```python
from build123d import *

# Parameters (mm, degrees)
F0_W      = 200
F0_H      = 100
F1_DEPTH  = 20
F3_DEPTH  = 10
F5_DEPTH  = 10
F6_R      = 45
F6_R_2    = 30
F7_DEPTH  = 10
F8_R      = 5
F9_DEPTH  = 25
F10_R     = 30
F11_DEPTH = 22


with BuildPart() as f1:
    # F0 (on Front) → F1 (new body)
    with BuildSketch(Plane.XZ):
        Rectangle(F0_W, F0_H)
    extrude(amount=F1_DEPTH)

    # F2 (on face) → F3 (cut)
    with BuildSketch(Plane.XZ.offset(20)):
        with BuildLine():
            Line((-72, 40), (-78, 40))
            ThreePointArc((-78, 40), (-86.485281, 36.485281), (-90, 28))
            Line((-90, 28), (-90, -28))
            ThreePointArc((-90, -28), (-86.485281, -36.485281), (-78, -40))
            Line((-78, -40), (-72, -40))
            ThreePointArc((-72, -40), (-63.514719, -36.485281), (-60, -28))
            Line((-60, -28), (-60, 28))
            ThreePointArc((-60, 28), (-63.514719, 36.485281), (-72, 40))
        make_face()
    extrude(amount=-F3_DEPTH, mode=Mode.SUBTRACT)

    # F4 (on face) → F5 (join)
    with BuildSketch(Plane.XZ.offset(20)):
        with BuildLine():
            Line((-38, -48), (43.029173, -48))
            ThreePointArc((43.029173, -48), (47.621583, -47.086468), (51.514773, -44.484963))
            Line((51.514773, -44.484963), (85.390988, -10.606203))
            ThreePointArc((85.390988, -10.606203), (89.783988, 0), (85.390988, 10.606203))
            Line((85.390988, 10.606203), (51.514773, 44.484963))
            ThreePointArc((51.514773, 44.484963), (47.621583, 47.086468), (43.029173, 48))
            Line((43.029173, 48), (-38, 48))
            ThreePointArc((-38, 48), (-45.071068, 45.071068), (-48, 38))
            Line((-48, 38), (-48, -38))
            ThreePointArc((-48, -38), (-45.071068, -45.071068), (-38, -48))
        make_face()
    extrude(amount=F5_DEPTH)

    # F6 (on face) → F7 (join)
    with BuildSketch(Plane.XZ.offset(30)):
        Circle(F6_R)
        Circle(F6_R_2, mode=Mode.SUBTRACT)
    extrude(amount=F7_DEPTH)

    # F8 (on face) → F9 (cut)
    with BuildSketch(Plane.XZ.offset(40)):
        with Locations((-37.533723, 0.141637)):
            Circle(F8_R)
        with Locations((36.967181, 0.42491)):
            Circle(F8_R)
        with Locations((0, 37.5)):
            Circle(F8_R)
        with Locations((0.424909, -37.250452)):
            Circle(F8_R)
    extrude(amount=-F9_DEPTH, mode=Mode.SUBTRACT)

    # F10 (on face) → F11 (cut)
    with BuildSketch(Plane.XZ.offset(30)):
        Circle(F10_R)
    extrude(amount=-F11_DEPTH, mode=Mode.SUBTRACT)


solid = f1.part
```
Geometry: final body of the model. Coordinates: model frame, mm. A direction names the side the tool comes from. Give positions to 0.01 mm unless a question says otherwise; leave off trailing zeros. Loops run counter-clockwise (first coordinate to the right, second up) from the corner with the lowest first, then second, coordinate; pieces in that order, holes last. Notation, with made-up numbers: (72.5, -27) - (111.5, -27) arc R33 cw to (111.5, 11) - close; hole circle Ø1 at (-10, -15.75). An arc over 180 degrees is marked (long way). Answer as CSV lines item,"result". Start each with the question number.
(1) Mould query, pull axis X, two halves, no side actions, for faces 4 (the face through (0, -8, 0)), 5 (the face through (-44.99, -24.93, 45.15)), 6 (the face through (2, -25, -48)). Classes: +X half, -X half, draft (parallel to the pull), parting line (faces both ways), or undercut.
(2) Section query D-D (x = 22). Output: boundary loops of the cut face in (y, z), and give its area (3 significant figures).
(3) Section query C-C (x = 0). Output: boundary loops of the cut face in (y, z), and give its area (3 significant figures).
(4) Ray query, line 1 along Z through (x, y) = (0, -23); line 2 along X through (y, z) = (-19.5, 27); line 3 along X through (y, z) = (-19, 25.5). Return the intervals inside material, ascending. Write a range as [from, to].
(5) Pin query (flat end, axial travel): P1, Ø10, axis at y = -29, z = 13.5, coming from the -X side; P2, Ø6, axis at x = 0, z = 37.5, coming from the -Y side. Return the tip coordinate at first contact, or that it passes through.
(6) Section query A-A (z = 8.5). Output: boundary loops of the cut face in (x, y).
(7) Reachability of faces 1 (the face through (0, -15, -37)), 2 (the face through (47.68, -24.93, 47.06)), 3 (the face through (3, -25, 48)) from +Z, -Z, +X, -X, +Y, -Y: full face, straight path, thin tool, end or side. Return the list, or none.
(8) Section query B-B (y = -34.5). Output: boundary loops of the cut face in (x, z).
Worked answers:
1,face 4,"undercut"
1,face 5,"-X half"
1,face 6,"draft"
2,outline,"(-40, -39.26) - (-30, -39.26) - (-30, -48) - (-20, -48) - (-20, -50) - (0, -50) - (0, 50) - (-20, 50) - (-20, 48) - (-30, 48) - (-30, 39.26) - (-40, 39.26) - (-40, 20.4) - (-8, 20.4) - (-8, -20.4) - (-40, -20.4) - close"
2,area,"2,440 mm^2"
3,outline,"(-40, -45) - (-30, -45) - (-30, -48) - (-20, -48) - (-20, -50) - (0, -50) - (0, 50) - (-20, 50) - (-20, 48) - (-30, 48) - (-30, 45) - (-40, 45) - (-40, 42.5) - (-15, 42.5) - (-15, 32.5) - (-40, 32.5) - (-40, 30) - (-8, 30) - (-8, -30) - (-40, -30) - (-40, -32.27) - (-15, -32.27) - (-15, -42.23) - (-40, -42.23) - close"
3,area,"1,440 mm^2"
4,line 1,"z = [-48, -42.23], [-32.27, -30], [30, 32.5], [42.5, 48]"
4,line 2,"x = [-100, -90], [-60, -13.08], [13.08, 100]"
4,line 3,"x = [-100, -90], [-60, -15.8], [15.8, 100]"
5,P1,"stops at x = -48"
5,P2,"stops at y = -15"
6,outline,"(-100, -20) - (-90, -20) - (-90, -10) - (-60, -10) - (-60, -20) - (-48, -20) - (-48, -30) - (-44.19, -30) - (-44.19, -40) - (-28.77, -40) - (-28.77, -8) - (28.77, -8) - (28.77, -40) - (44.19, -40) - (44.19, -30) - (87.14, -30) - (87.14, -20) - (100, -20) - (100, 0) - (-100, 0) - close"
7,face 1,"-Y"
7,face 2,"+Z, +X, -Y"
7,face 3,"+Z, +X, -X, -Y"
8,outline,"circle Ø90 at (0, 0); hole circle Ø10 at (-37.53, 0.14); hole circle Ø60 at (0, 0); hole circle Ø10 at (0, 37.5); hole circle Ø10 at (0.42, -37.25); hole circle Ø10 at (36.97, 0.42)"
